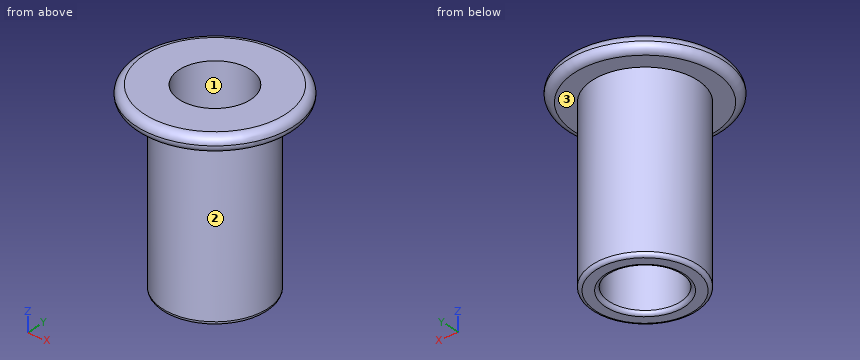
```python
from build123d import *

# Parameters (mm, degrees)
SKETCH_1_R      = 2.95
SKETCH_1_R_2    = 2
EXTRUDE_1_DEPTH = 9.6
EXTRUDE_START   = 0.9
SKETCH_2_R      = 4.4
SKETCH_2_R_2    = 2
EXTRUDE_2_DEPTH = 0.9
FILLET_1_R      = 0.45
FILLET_2_R      = 0.2


with BuildPart() as part:
    # 草图1 → 凸台-拉伸1 (new body)
    with BuildSketch(Plane.XY):
        Circle(SKETCH_1_R)
        Circle(SKETCH_1_R_2, mode=Mode.SUBTRACT)
    extrude(amount=-EXTRUDE_1_DEPTH)

    # 草图2 → 凸台-拉伸2 (add)
    with BuildSketch(Plane.XY.offset(EXTRUDE_START)):
        Circle(SKETCH_2_R)
        Circle(SKETCH_2_R_2, mode=Mode.SUBTRACT)
    extrude(amount=-EXTRUDE_2_DEPTH)

    # 圆角1
    fillet_1_edges = [part.edges().sort_by_distance(p)[0] for p in [
        (-4.4, 0, 0),
        (-4.4, 0, 0.9),
    ]]
    fillet(fillet_1_edges, radius=FILLET_1_R - 0.0001)  # a hair under: the kernel refuses the full size

    # 圆角2
    fillet_2_edges = [part.edges().sort_by_distance(p)[0] for p in [
        (-2.95, 0, -9.6),
        (-2, 0, -9.6),
    ]]
    fillet(fillet_2_edges, radius=FILLET_2_R)


solid = part.part
```
CAD build for the part. Positions are in the model's coordinates, mm. Face numbers are marked on the shaded views. Round coordinates to 2 decimals unless told otherwise and drop trailing zeros. Loops run counter-clockwise (first coordinate to the right, second up) from the corner with the lowest first, then second, coordinate; pieces in that order, holes last. Notation, with made-up numbers: M -40,27 L 2,27 A21 cw 2,44 Z; hole C 16.5,-36.75 d2. An arc over 180 degrees is marked long. Return JSON: item names as keys, results as strings. Group by question number.
(1) Wall check: probe 1 along Y at (x, z) = (0, -2); probe 2 along Z at (x, y) = (-0.25, -3); probe 3 along X at (y, z) = (-0.5, -3). Give the ranges that are in metal, low to high. Write a range as [from, to].
(2) Saw through at C-C, the plane z = -1. List the corners of the cut face in (x, y).
(3) Drop flat-ended pins along their axis: P1, Ø1.5, axis at x = 0, y = 0.5, coming from the -Z side; P2, Ø5, axis at x = -1.5, z = -7.5, coming from the -Y side; P3, Ø1.5, axis at y = -1, z = -3, coming from the +X side; P4, Ø1, axis at x = 3.5, y = 0.5, coming from the -Z side. Give the stop position or say it passes through.
(4) Mould opens along Y. For the marked faces 1, 2 and 3 say: +Y half, -Y half, draft (parallel to the pull), parting line (faces both ways), or undercut.
Answer list:
{
 "1": {"probe 1": "[-2.95, -2], [2, 2.95]", "probe 2": "[0, 0.9]", "probe 3": "[-2.91, -1.94], [1.94, 2.91]"},
 "2": {"outline": "C 0,0 d5.9; hole C 0,0 d4"},
 "3": {"P1": "through", "P2": "y = -2.95", "P3": "x = 2.94", "P4": "z = 0"},
 "4": {"face 1": "undercut", "face 2": "parting line", "face 3": "draft"}
}
